from build123d import *

# Parameters (mm, degrees)
F1_DEPTH = 44.45
F3_W     = 38.1
F3_H     = 50.8
F4_DEPTH = 76.2
F6_W     = 38.1
F6_H     = 50.8
F7_DEPTH = 76.2


with BuildPart() as f1:
    # F0 (on Right) → F1 (new body, symmetric)
    with BuildSketch(Plane.YZ):
        Polygon((-182.88, 406.4), (-285.496, 406.4), (183.774299, -406.4), (286.390299, -406.4), align=None)
    extrude(amount=F1_DEPTH, both=True)

    # F3 (on offset) → F4 (cut)
    with BuildSketch(Plane.XZ.offset(272.288)):
        with Locations((0, 361.95)):
            Rectangle(F3_W, F3_H)
    extrude(amount=-F4_DEPTH, mode=Mode.SUBTRACT)

    # F6 (on offset) → F7 (cut)
    with BuildSketch(Plane.XZ.offset(-101.6)):
        with Locations((0, -177.8)):
            Rectangle(F6_W, F6_H)
    extrude(amount=F7_DEPTH, mode=Mode.SUBTRACT)


solid = f1.part
Design review of the part built by this model. Coordinates are the model's own, in mm. A direction names the side the tool comes from. Give positions to 0.01 mm unless a question says otherwise; leave off trailing zeros. Loops run counter-clockwise (first coordinate to the right, second up) from the corner with the lowest first, then second, coordinate; pieces in that order, holes last. Notation, with made-up numbers: (14.25, 4) -> (47.25, 4) arc R12 ccw to (47.25, 14) -> close; hole circle Ø1 at (-19, -4). An arc over 180 degrees is marked (long way). One line per question, with ' | ' between items. Start each with the question number.
(1) We need section D-D (y = -37). State the section outline as (x, z) points.
(2) For line 1 (Z direction, x = 13.5, y = 89.5); line 2 (Z direction, x = -20, y = -89); line 3 (Z direction, x = -2, y = -92), list the stretches that pass through material, from the lowest coordinate up.
(3) Draft analysis for pull direction X (two halves, no side actions). For faces 4 (the face through (-19.05, -226, 362)), 5 (the face through (-44.45, -1, 2)), 6 (the face through (0, 70, -152.4)), 7 (the face through (0.622, -54.146, 5.69)), state which applies: +X half, -X half, draft (parallel to the pull), parting line (faces both ways), or undercut.
(4) We need section B-B (z = -188.5). State the section outline as (x, y) points, and give its area (3 significant figures).
(5) We need section A-A (x = -6). State the section outline as (y, z) points.
(6) Insertion check: P1, Ø1.1, axis at x = 4, z = 385, coming from the +Y side; P2, Ø10.5, axis at x = -7.5, y = 79.5, coming from the +Z side; P3, Ø4, axis at x = 13, y = -151, coming from the -Z side. Each pin has a flat end and moves straight along its axis. Give the tip position at first contact, or say it passes through.
(7) For faces 1 (the face through (0, 84, -203.2)), 2 (the face through (44.45, -1, 2)), 3 (the face through (19.05, -226, 362)), list the 3-axis set-ups (+Z, -Z, +X, -X, +Y, -Y) from which the entire face can be reached by the end or side of a thin tool; tool diameter is ignored.
(8) We need section C-C (y = 247). State the section outline as (x, z) points, and give its area (3 significant figures).
The answers:
1) outline: (-44.45, -24.01) -> (44.45, -24.01) -> (44.45, 153.73) -> (-44.45, 153.73) -> close
2) line 1: z = -243.11 to -203.2, -152.4 to -65.38 | line 2: z = 66.06 to 243.8 | line 3: z = 71.26 to 248.99
3) face 4: undercut | face 5: -X half | face 6: undercut | face 7: draft
4) outline: (-44.45, 57.97) -> (-19.05, 57.97) -> (-19.05, 101.6) -> (19.05, 101.6) -> (19.05, 57.97) -> (44.45, 57.97) -> (44.45, 160.59) -> (-44.45, 160.59) -> close | area: 7,460 mm^2
5) outline: (-285.5, 406.4) -> (-272.29, 383.52) -> (-272.29, 387.35) -> (-196.09, 387.35) -> (-196.09, 336.55) -> (-245.17, 336.55) -> (37.13, -152.4) -> (101.6, -152.4) -> (101.6, -203.2) -> (66.46, -203.2) -> (183.77, -406.4) -> (286.39, -406.4) -> (-182.88, 406.4) -> close
6) P1: stops at y = -170.21 | P2: stops at z = -38.96 | P3: stops at z = 169.98
7) face 1: -Y | face 2: +Z, -Z, +X, +Y, -Y | face 3: none
8) outline: (-44.45, -406.4) -> (44.45, -406.4) -> (44.45, -338.17) -> (-44.45, -338.17) -> close | area: 6,070 mm^2
